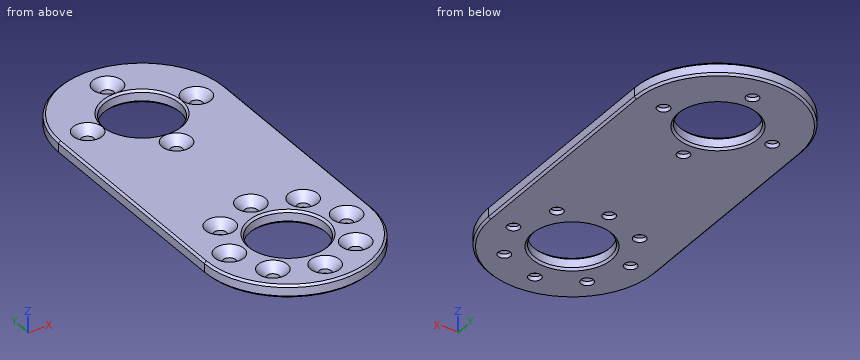
```python
from build123d import *

# Parameters (mm, degrees)
ESQUISSE1_R      = 9
ESQUISSE1_R_2    = 1.5
EXTRUSION1_DEPTH = 3
CHANFREIN1_SIZE  = 2
CHANFREIN2_SIZE  = 0.5


with BuildPart() as part:
    # Esquisse1 → Extrusion1 (new body)
    with BuildSketch(Plane.XY):
        with BuildLine():
            Line((0, 0), (0, 55))
            ThreePointArc((0, 55), (20, 75), (40, 55))
            Line((40, 55), (40, 0))
            ThreePointArc((40, 0), (20, -20), (0, 0))
        make_face()
        with Locations((20, 55)):
            Circle(ESQUISSE1_R, mode=Mode.SUBTRACT)
        with Locations((20, 0)):
            Circle(ESQUISSE1_R, mode=Mode.SUBTRACT)
        with Locations((20, 68)):
            Circle(ESQUISSE1_R_2, mode=Mode.SUBTRACT)
        with Locations(Location((20, 42, 0), (0, 0, 180))):
            Circle(ESQUISSE1_R_2, mode=Mode.SUBTRACT)
        with Locations((7, 55)):
            Circle(ESQUISSE1_R_2, mode=Mode.SUBTRACT)
        with Locations(Location((33, 55, 0), (0, 0, 180))):
            Circle(ESQUISSE1_R_2, mode=Mode.SUBTRACT)
        with Locations((10.100505063, 9.899494937)):
            Circle(ESQUISSE1_R_2, mode=Mode.SUBTRACT)
        with Locations((6, 0)):
            Circle(ESQUISSE1_R_2, mode=Mode.SUBTRACT)
        with Locations((10.100505063, -9.899494937)):
            Circle(ESQUISSE1_R_2, mode=Mode.SUBTRACT)
        with Locations((20, -14)):
            Circle(ESQUISSE1_R_2, mode=Mode.SUBTRACT)
        with Locations((29.899494937, -9.899494937)):
            Circle(ESQUISSE1_R_2, mode=Mode.SUBTRACT)
        with Locations((34, 0)):
            Circle(ESQUISSE1_R_2, mode=Mode.SUBTRACT)
        with Locations((29.899494937, 9.899494937)):
            Circle(ESQUISSE1_R_2, mode=Mode.SUBTRACT)
        with Locations((20, 14)):
            Circle(ESQUISSE1_R_2, mode=Mode.SUBTRACT)
    extrude(amount=EXTRUSION1_DEPTH)

    # Chanfrein1
    chanfrein1_edges = [part.edges().sort_by_distance(p)[0] for p in [
        (18.5, 68, 3),
        (21.5, 42, 3),
        (5.5, 55, 3),
        (34.5, 55, 3),
        (8.600505063, 9.899494937, 3),
        (4.5, 0, 3),
        (8.600505063, -9.899494937, 3),
        (18.5, -14, 3),
        (28.399494937, -9.899494937, 3),
        (32.5, 0, 3),
        (28.399494937, 9.899494937, 3),
        (18.5, 14, 3),
    ]]
    chamfer(chanfrein1_edges, length=CHANFREIN1_SIZE)

    # Chanfrein2
    chanfrein2_edges = [part.edges().sort_by_distance(p)[0] for p in [
        (20, 75, 3),
        (11, 55, 0),
        (11, 55, 3),
        (0, 27.5, 3),
        (11, 0, 0),
        (11, 0, 3),
        (20, -20, 3),
        (0, 27.5, 0),
        (20, 75, 0),
        (40, 27.5, 0),
        (20, -20, 0),
        (40, 27.5, 3),
    ]]
    chamfer(chanfrein2_edges, length=CHANFREIN2_SIZE - 0.0001)  # a hair under: the kernel refuses the full size


solid = part.part
```
The listing builds one solid part. Answer for the finished solid, in the listing's coordinates (mm). Coordinates: 2 decimals unless noted, no trailing zeros. Loops run counter-clockwise (first coordinate to the right, second up) from the corner with the lowest first, then second, coordinate; pieces in that order, holes last. Notation, with made-up numbers: (8, 10) - (49, 10) arc R16 ccw to (49, 24) - close; hole circle Ø3 at (-36, 10.25). An arc over 180 degrees is marked (long way). Write item = value, one per line.
1) Find the intervals of material crossed by line 1 along Y through (x, z) = (16, 1.1); line 2 along Y through (x, z) = (14.5, 1.5); line 3 along X through (y, z) = (-1.5, 2.5), in increasing order.
Responses:
line_1 = -19.6 to -8.06, 8.06 to 46.94, 63.06 to 74.6
line_2 = -19.23 to -7.12, 7.12 to 47.88, 62.12 to 74.23
line_3 = 0.06 to 3.4, 8.6 to 11.13, 28.87 to 31.4, 36.6 to 39.94
2) Each of these flat-tipped pins is pushed along its axis until it touches: P1, Ø2.5, axis at x = 20, y = 14, coming from the -Z side; P2, Ø3.5, axis at x = 29.9, y = -9.9, coming from the +Z side; P3, Ø4, axis at x = 10.1, y = 9.9, coming from the +Z side; P4, Ø1, axis at y = 56.5, z = 2.5, coming from the +X side (3 decimals). Where does it stop, or does it pass through?
Responses:
P1 = through
P2 = 1.25
P3 = 1.5
P4 = 39.975
3) Section A-A (y = 42) is taken. Determine the outline of the cut face in (x, z).
Responses:
outline = (0, 0.5) - (0.5, 0) - (18.5, 0) - (18.5, 1) - (16.5, 3) - (0.5, 3) - (0, 2.5) - close; (21.5, 0) - (39.5, 0) - (40, 0.5) - (40, 2.5) - (39.5, 3) - (23.5, 3) - (21.5, 1) - close
4) Section B-B (z = 2) is taken. Count the separate pieces of the cut face and the enclosed holes in it, plus the area to 3 significant figures.
Responses:
separate_pieces = 1
enclosed_holes = 14
area = 2,710 mm^2
